Geometry check sheet. Reference: drawing and pictorial views, mm from the part's lowest x, y, z. A direction names the side the tool comes from. Round coordinates to 2 decimals unless told otherwise and drop trailing zeros. Loops run counter-clockwise (first coordinate to the right, second up) from the corner with the lowest first, then second, coordinate; pieces in that order, holes last. Notation, with made-up numbers: (-26.5, -17) -> (15.5, -17) arc R29 cw to (15.5, 19) -> close; hole circle Ø8 at (16, 65). An arc over 180 degrees is marked (long way). Use one line per item in the form item = value. Start each with the question number.
(1) Material ranges on probe 1 along X at (y, z) = (6, 24); probe 2 along Z at (x, y) = (52.5, 5.75); probe 3 along X at (y, z) = (6.5, 31.5), recorded low to high. Write a range as [from, to].
(2) Set-up check for the marked faces 4 and 5: record each of +Z, -Z, +X, -X, +Y, -Y from which the full face is reachable in a straight line by a thin tool's end or side.
(3) Go/stop test with a flat-tipped pin: pin 1 (4.5 mm diameter, centred on x = 77, z = 26.5, fed in from -Y). Record where the tip stops, or that it passes through.
(4) Draft check along X on the marked faces 1, 2 and 3. Enter one of: released by +X, released by -X, zero draft, split by the parting line, or undercut.
(5) Sectioned sample at C-C (z = 30). Record the cut outline in (x, y).
(6) Sectioned sample at D-D (x = 82). Record the cut outline in (y, z), and give its area (3 significant figures).
(7) Sectioned sample at B-B (x = 27.5). Record the cut outline in (y, z), and give its area (3 significant figures).
(8) Sectioned sample at A-A (y = 8.5). Record the cut outline in (x, z).
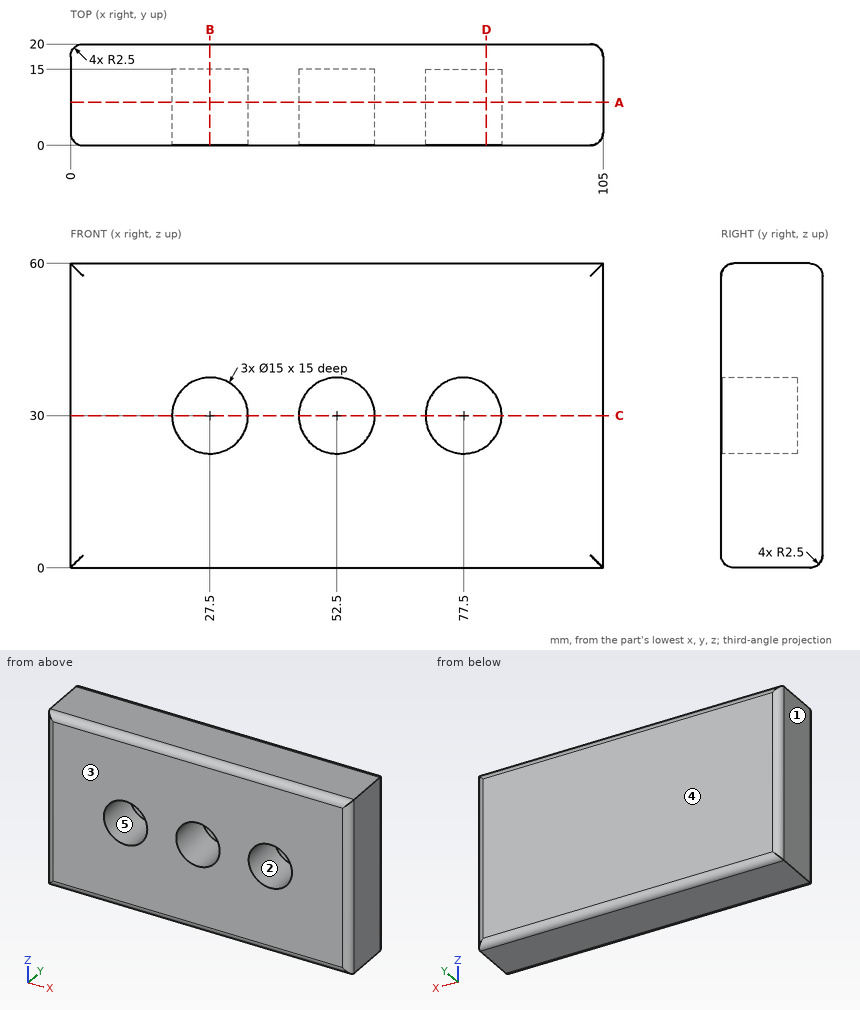
Checks:
q1.probe_1 = [0, 23], [32, 48], [57, 73], [82, 105]
q1.probe_2 = [0, 22.5], [37.5, 60]
q1.probe_3 = [0, 20.15], [34.85, 45.15], [59.85, 70.15], [84.85, 105]
q2.face_4 = +Z, -Z, +X, -X, +Y
q2.face_5 = -Y
q3.pin_1 = 15
q4.face_1 = released by -X
q4.face_2 = undercut
q4.face_3 = zero draft
q5.outline = (0, 2.5) arc R2.5 ccw to (2.5, 0) -> (20, 0) -> (20, 15) -> (35, 15) -> (35, 0) -> (45, 0) -> (45, 15) -> (60, 15) -> (60, 0) -> (70, 0) -> (70, 15) -> (85, 15) -> (85, 0) -> (102.5, 0) arc R2.5 ccw to (105, 2.5) -> (105, 17.5) arc R2.5 ccw to (102.5, 20) -> (2.5, 20) arc R2.5 ccw to (0, 17.5) -> close
q6.outline = (0, 2.5) arc R2.5 ccw to (2.5, 0) -> (17.5, 0) arc R2.5 ccw to (20, 2.5) -> (20, 57.5) arc R2.5 ccw to (17.5, 60) -> (2.5, 60) arc R2.5 ccw to (0, 57.5) -> (0, 36) -> (15, 36) -> (15, 24) -> (0, 24) -> close
q6.area = 1,010 mm2
q7.outline = (0, 2.5) arc R2.5 ccw to (2.5, 0) -> (17.5, 0) arc R2.5 ccw to (20, 2.5) -> (20, 57.5) arc R2.5 ccw to (17.5, 60) -> (2.5, 60) arc R2.5 ccw to (0, 57.5) -> (0, 37.5) -> (15, 37.5) -> (15, 22.5) -> (0, 22.5) -> close
q7.area = 970 mm2
q8.outline = (0, 0) -> (105, 0) -> (105, 60) -> (0, 60) -> close; hole circle Ø15 at (27.5, 30); hole circle Ø15 at (52.5, 30); hole circle Ø15 at (77.5, 30)
